Source: CAD feature listing. Evaluate the final solid. Frame: model axes, mm. Coordinates: 2 decimals unless noted, no trailing zeros. Loops run counter-clockwise (first coordinate to the right, second up) from the corner with the lowest first, then second, coordinate; pieces in that order, holes last. Notation, with made-up numbers: (76.5, -12) -> (89.5, -12) arc R19 ccw to (89.5, 4) -> close; hole circle Ø9 at (77.25, -24.5). An arc over 180 degrees is marked (long way). Answer as a JSON object with one key per item and string values. Group by question number.
from build123d import *

# Parameters (mm, degrees)
PAD_DEPTH       = 5
SKETCH001_R     = 1.5
SKETCH001_R_2   = 1.6
SKETCH001_R_3   = 2.1
POCKET_DEPTH    = 5.001
SKETCH002_R     = 2.55
POCKET001_DEPTH = 5.001


with BuildPart() as part:
    # Sketch → Pad (new body)
    with BuildSketch(Plane.XY):
        Polygon((-180, 375), (180, 375), (185, 370), (185, 10), (180, 5), (-34, 5), (-39, 10), (-58, 10), (-63, 5), (-144, 5), (-148, 9), (-156, 9), (-160, 5), (-180, 5), (-185, 10), (-185, 370), align=None)
        Polygon((-135, 56.5), (-135, 330), (-130, 335), (130, 335), (135, 330), (135, 56.5), (130, 51.5), (112, 51.5), (102, 41.5), (97, 41.5), (92, 36.5), (78, 36.5), (73, 41.5), (25, 41.5), (5, 21.5), (-5, 21.5), (-25, 41.5), (-73, 41.5), (-78, 36.5), (-92, 36.5), (-97, 41.5), (-102, 41.5), (-112, 51.5), (-130, 51.5), align=None, mode=Mode.SUBTRACT)
    extrude(amount=PAD_DEPTH)

    # Sketch001 → Pocket (cut, through all)
    with BuildSketch(Plane.XY.offset(5)):
        with Locations((-175, 364.8)):
            Circle(SKETCH001_R)
        with Locations((-155, 364.8)):
            Circle(SKETCH001_R)
        with Locations((155, 364.8)):
            Circle(SKETCH001_R)
        with Locations((175, 364.8)):
            Circle(SKETCH001_R)
        with Locations((-175, 44.8)):
            Circle(SKETCH001_R)
        with Locations((-155, 44.8)):
            Circle(SKETCH001_R)
        with Locations((155, 44.8)):
            Circle(SKETCH001_R)
        with Locations((175, 44.8)):
            Circle(SKETCH001_R)
        with Locations((-32, 18)):
            Circle(SKETCH001_R_2)
        with Locations((-32, 9)):
            Circle(SKETCH001_R_2)
        with Locations((-65, 18)):
            Circle(SKETCH001_R_2)
        with Locations((-65, 9)):
            Circle(SKETCH001_R_2)
        with Locations((45, 18)):
            Circle(SKETCH001_R_2)
        with Locations((45, 9)):
            Circle(SKETCH001_R_2)
        with Locations((-65, 25)):
            Circle(SKETCH001_R_2)
        with Locations((-65, 35)):
            Circle(SKETCH001_R_2)
        with Locations((-165, 24.8)):
            Circle(SKETCH001_R)
        with Locations((-159, 12)):
            Circle(SKETCH001_R_2)
        with Locations((-145, 12)):
            Circle(SKETCH001_R_2)
        with Locations((165, 24.8)):
            Circle(SKETCH001_R)
        with Locations((146, 12)):
            Circle(SKETCH001_R_2)
        with Locations((158, 12)):
            Circle(SKETCH001_R_2)
        with Locations((-142.1, 72.8)):
            Circle(SKETCH001_R)
        with Locations((-138, 104.8)):
            Circle(SKETCH001_R)
        with Locations((-180.1, 72.8)):
            Circle(SKETCH001_R)
        with Locations((-181.3, 186.1)):
            Circle(SKETCH001_R)
        with Locations((-180.1, 166.8)):
            Circle(SKETCH001_R)
        with Locations((-181.3, 104.8)):
            Circle(SKETCH001_R)
        with Locations((-142.1, 166.8)):
            Circle(SKETCH001_R)
        with Locations((-138, 179.7)):
            Circle(SKETCH001_R)
        with Locations((-170, 252.8)):
            Circle(SKETCH001_R)
        with Locations((-181.5, 274.3)):
            Circle(SKETCH001_R)
        with Locations((-170, 295.8)):
            Circle(SKETCH001_R)
        with Locations((-138.5, 274.3)):
            Circle(SKETCH001_R)
        with Locations((148.4, 210)):
            Circle(SKETCH001_R_3)
        with Locations((148.4, 93)):
            Circle(SKETCH001_R_3)
    extrude(amount=-POCKET_DEPTH, mode=Mode.SUBTRACT)

    # Sketch002 → Pocket001 (cut, through all)
    with BuildSketch(Plane.XY.offset(5)):
        with Locations((-133.6, 33.1)):
            Circle(SKETCH002_R)
        with Locations((-110.4, 33.1)):
            Circle(SKETCH002_R)
        with Locations((-96.6, 33.1)):
            Circle(SKETCH002_R)
        with Locations((-73.4, 33.1)):
            Circle(SKETCH002_R)
        with Locations((-73.4, 9.9)):
            Circle(SKETCH002_R)
        with Locations((-96.6, 9.9)):
            Circle(SKETCH002_R)
        with Locations((-110.4, 9.9)):
            Circle(SKETCH002_R)
        with Locations((-133.6, 9.9)):
            Circle(SKETCH002_R)
        with Locations((73.4, 33.1)):
            Circle(SKETCH002_R)
        with Locations((96.6, 33.1)):
            Circle(SKETCH002_R)
        with Locations((110.4, 33.1)):
            Circle(SKETCH002_R)
        with Locations((133.6, 33.1)):
            Circle(SKETCH002_R)
        with Locations((133.6, 9.9)):
            Circle(SKETCH002_R)
        with Locations((110.4, 9.9)):
            Circle(SKETCH002_R)
        with Locations((96.6, 9.9)):
            Circle(SKETCH002_R)
        with Locations((73.4, 9.9)):
            Circle(SKETCH002_R)
    extrude(amount=-POCKET001_DEPTH, mode=Mode.SUBTRACT)


solid = part.part
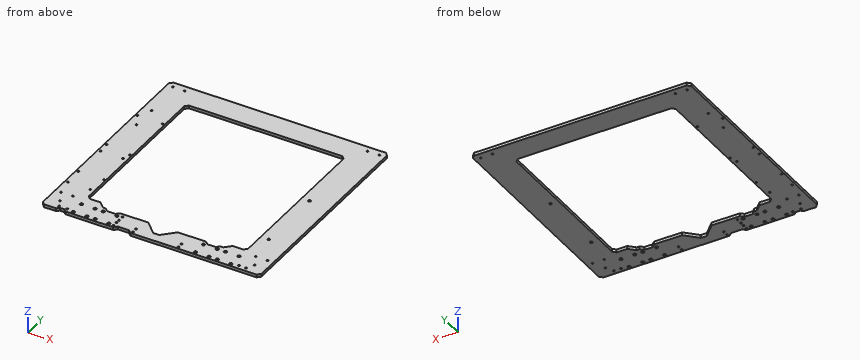
1. Pin query (flat end, axial travel): pin 1 Ø2.5 at (x, z) = (-153, 2) entering from -Y. Return the tip coordinate at first contact, or that it passes through.
2. Ray query, L1, parallel to Y at x = 148.4, z = 3.7; L2, parallel to X at y = 295.5, z = 3.4; L3, parallel to X at y = 72.8, z = 1.95. Return the intervals inside material, ascending.
3. Section query C-C on z = 1.45. State how many separate pieces and enclosed holes the cut face has, then the cut area to 3 significant figures.
4. Section query A-A on x = 10. Return loops of the section in (y, z).
5. Section query B-B on y = 266.5. Return loops of the section in (x, z), then the cut area to 3 significant figures.
Solved:
{
 "1": {"pin 1": "y = 9"},
 "2": {"L1": "5 to 90.9, 95.1 to 207.9, 212.1 to 375", "L2": "-185 to -171.47, -168.53 to -135, 135 to 185", "L3": "-185 to -181.6, -178.6 to -143.6, -140.6 to -135, 135 to 185"},
 "3": {"separate pieces": "1", "enclosed holes": "53", "area": "56,700 mm^2"},
 "4": {"outline": "(5, 0) -> (26.5, 0) -> (26.5, 5) -> (5, 5) -> close; (335, 0) -> (375, 0) -> (375, 5) -> (335, 5) -> close"},
 "5": {"outline": "(-185, 0) -> (-135, 0) -> (-135, 5) -> (-185, 5) -> close; (135, 0) -> (185, 0) -> (185, 5) -> (135, 5) -> close", "area": "500 mm^2"}
}
